from build123d import *

# Parameters (mm, degrees)
SKETCH1_W      = 17
SKETCH1_H      = 17
EXTRUDE1_DEPTH = 374
FILLET2_R      = 2
SKETCH2_W      = 13
SKETCH2_H      = 13
EXTRUDE2_DEPTH = 375
FILLET3_R      = 2
SKETCH3_R      = 2.5
EXTRUDE3_DEPTH = 18


with BuildPart() as part:
    # Sketch1 → Extrude1 (new body)
    with BuildSketch(Plane.XY):
        with Locations((-39.634997969, 15.034639228)):
            Rectangle(SKETCH1_W, SKETCH1_H)
    extrude(amount=EXTRUDE1_DEPTH)

    # Fillet2
    fillet2_edges = [part.edges().sort_by_distance(p)[0] for p in [
        (-48.134997969, 23.534639228, 187),
        (-31.134997969, 23.534639228, 187),
        (-31.134997969, 6.534639228, 187),
        (-48.134997969, 6.534639228, 187),
    ]]
    fillet(fillet2_edges, radius=FILLET2_R)

    # Sketch2 → Extrude2 (cut, through all)
    with BuildSketch(Plane.XY.offset(374)):
        with Locations((-39.634997969, 15.034639228)):
            Rectangle(SKETCH2_W, SKETCH2_H)
    extrude(amount=-EXTRUDE2_DEPTH, mode=Mode.SUBTRACT)

    # Fillet3
    fillet3_edges = [part.edges().sort_by_distance(p)[0] for p in [
        (-46.134997969, 8.534639228, 187),
        (-46.134997969, 21.534639228, 187),
        (-33.134997969, 21.534639228, 187),
        (-33.134997969, 8.534639228, 187),
    ]]
    fillet(fillet3_edges, radius=FILLET3_R)

    # Sketch3 → Extrude3 (cut, through all)
    with BuildSketch(Plane(origin=(-31.134997969, 0, 0), x_dir=(0, 0, -1), z_dir=(1, 0, 0))):
        with Locations((-369, 15.034639228)):
            Circle(SKETCH3_R)
        with Locations((-354, 15.034639228)):
            Circle(SKETCH3_R)
        with Locations((-9, 15.034639228)):
            Circle(SKETCH3_R)
    extrude(amount=-EXTRUDE3_DEPTH, mode=Mode.SUBTRACT)


solid = part.part
Source: CAD feature listing. Evaluate the final solid. Frame: model axes, mm. A direction names the side the tool comes from. Round coordinates to 2 decimals unless told otherwise and drop trailing zeros. Write each loop counter-clockwise with the first axis right and the second up, starting at its lowest first coordinate (ties: lowest second). Pieces come first, ordered by that corner, then holes. Notation, with made-up numbers: (26, 22) - (83, 22) arc R25 ccw to (83, 48) - close; hole circle Ø10 at (32, -1.5). An arc over 180 degrees is marked (long way). Use CSV: the item, a comma, the result in double quotes. Start each with the question number.
(1) Cut plane A-A, the plane z = 301. Return loops of the section in (x, y) (3 decimals), and give its area (3 significant figures).
(2) First-contact query: pin 1 Ø1.5 at (x, y) = (-44.5, 12.5) entering from +Z. Flat tip, straight axial feed; report the tip coordinate or a pass-through.
(3) Mould query, pull axis X, two halves, no side actions, for faces 3 (the face through (-48.135, 15, 184)), 4 (the face through (-46.135, 15, 190)), 5 (the face through (-40, 21.535, 190)), 6 (the face through (-31.135, 15, 184)). Classes: pulls with the +X half, pulls with the -X half, needs draft (parallel to the pull), parting line crosses it, or undercut.
(4) Set-up query: faces 1 (the face through (-40, 6.535, 184)), 2 (the face through (-33.135, 15, 190)). Return all of +Z, -Z, +X, -X, +Y, -Y with unobstructed straight access to the full face (end or side cutting, diameter ignored); none if empty.
(5) Material intervals for probe 1 along X at (y, z) = (11.5, 217.5) (3 decimals); probe 2 along Y at (x, z) = (-40.5, 327.5); probe 3 along Z at (x, y) = (-47.25, 12.75), sorted ascending. Write a range as [from, to].
Geometry says:
1,outline,"(-48.135, 8.535) arc R2 ccw to (-46.135, 6.535) - (-33.135, 6.535) arc R2 ccw to (-31.135, 8.535) - (-31.135, 21.535) arc R2 ccw to (-33.135, 23.535) - (-46.135, 23.535) arc R2 ccw to (-48.135, 21.535) - close; hole (-46.135, 10.535) arc R2 ccw to (-44.135, 8.535) - (-35.135, 8.535) arc R2 ccw to (-33.135, 10.535) - (-33.135, 19.535) arc R2 ccw to (-35.135, 21.535) - (-44.135, 21.535) arc R2 ccw to (-46.135, 19.535) - close"
1,area,"120 mm²"
2,pin 1,"through"
3,face 3,"pulls with the -X half"
3,face 4,"undercut"
3,face 5,"undercut"
3,face 6,"pulls with the +X half"
4,face 1,"+Z, -Z, +X, -X, -Y"
4,face 2,"+Z, -Z"
5,probe 1,"[-48.135, -46.135], [-33.135, -31.135]"
5,probe 2,"[6.53, 8.53], [21.53, 23.53]"
5,probe 3,"[0, 7.98], [10.02, 352.98], [355.02, 367.98], [370.02, 374]"
